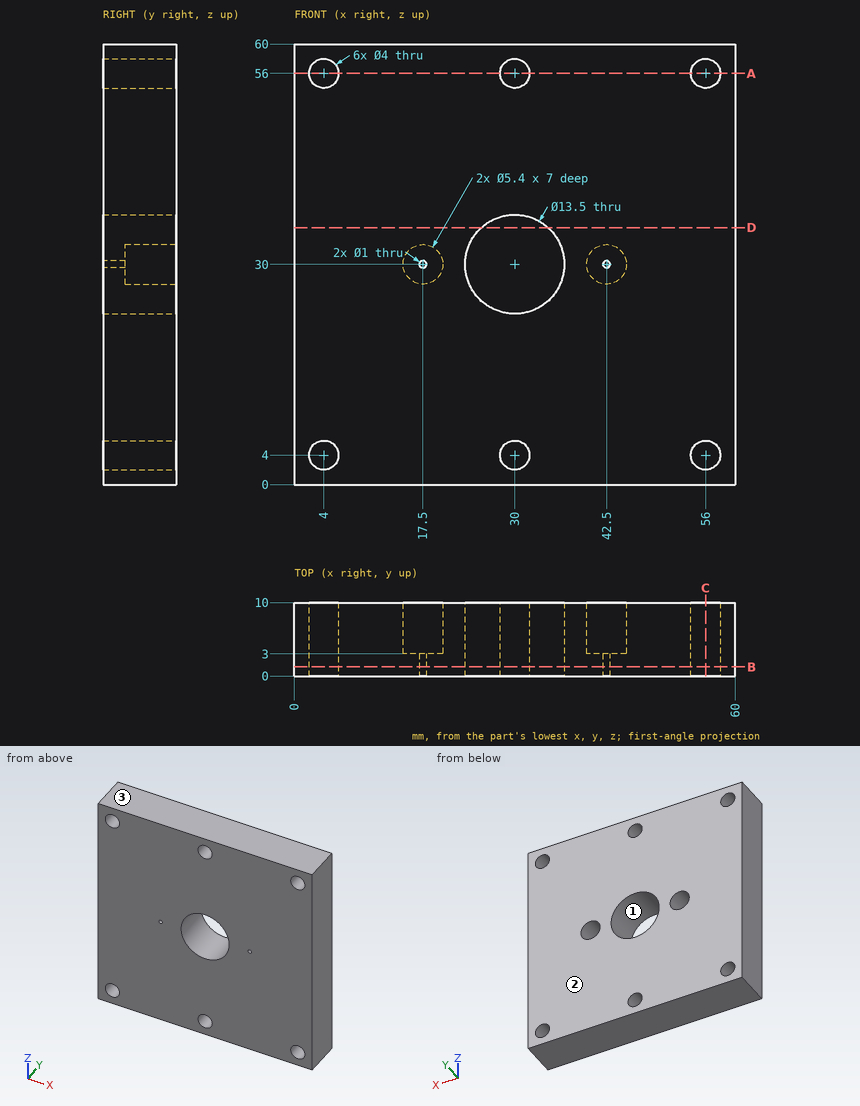
Could you check a few things on this drawing? It's one solid part, dimensions in mm from its lowest x, y, z. Round coordinates to 2 decimals unless told otherwise and drop trailing zeros. Loops run counter-clockwise (first coordinate to the right, second up) from the corner with the lowest first, then second, coordinate; pieces in that order, holes last. Notation, with made-up numbers: M 35.5,17.25 L 40.5,17.25 A12 cw 40.5,30.25 Z; hole C 15.25,-1.5 d1. An arc over 180 degrees is marked long. Write item = value, one per line. Start each with the question number.
(1) If we mould it in two halves opening along Z, with no side actions, what happens to the marked faces 1, 2 and 3? For each: released by +Z, released by -Z, zero draft, split by the parting line, or undercut.
(2) Suppose I cut it at C-C on x = 56. Write out the boundary of the cut face in (y, z), plus the area to 3 significant figures.
(3) I'm going to push flat-ended pins straight in: P1, Ø3.5, axis at x = 30, z = 56, coming from the -Y side (3 decimals); P2, Ø4.5, axis at x = 4, z = 56, coming from the -Y side; P3, Ø2.5, axis at x = 17, z = 30.5, coming from the +Y side. Where does each tip first touch, or does it pass through?
(4) Suppose I cut it at D-D on z = 35. Write out the boundary of the cut face in (x, y), plus the area to 3 significant figures.
(5) I need wall thicknesses on line 1 along Z through (x, y) = (30, 3); line 2 along X through (y, z) = (4, 56); line 3 along X through (y, z) = (5.75, 30). Which ranges of each line are inside material? Lowest first, please.
(6) Suppose I cut it at A-A on z = 56. Write out the boundary of the cut face in (x, y).
(7) Suppose I cut it at B-B on y = 1.25. Give the number of separate pieces and of enclosed holes in the cut face, plus the area to 3 significant figures.
Answer block:
q1.face_1 = undercut
q1.face_2 = zero draft
q1.face_3 = released by +Z
q2.outline = M 0,0 L 10,0 L 10,2 L 0,2 Z; M 0,6 L 10,6 L 10,54 L 0,54 Z; M 0,58 L 10,58 L 10,60 L 0,60 Z
q2.area = 520 mm²
q3.P1 = through
q3.P2 = 0
q3.P3 = 3
q4.outline = M 0,0 L 25.47,0 L 25.47,10 L 0,10 Z; M 34.53,0 L 60,0 L 60,10 L 34.53,10 Z
q4.area = 509 mm²
q5.line_1 = 0 to 2, 6 to 23.25, 36.75 to 54, 58 to 60
q5.line_2 = 0 to 2, 6 to 28, 32 to 54, 58 to 60
q5.line_3 = 0 to 14.8, 20.2 to 23.25, 36.75 to 39.8, 45.2 to 60
q6.outline = M 0,0 L 2,0 L 2,10 L 0,10 Z; M 6,0 L 28,0 L 28,10 L 6,10 Z; M 32,0 L 54,0 L 54,10 L 32,10 Z; M 58,0 L 60,0 L 60,10 L 58,10 Z
q7.separate_pieces = 1
q7.enclosed_holes = 9
q7.area = 3,380 mm²
